Source: CAD feature listing. Evaluate the final solid. Frame: model axes, mm. A direction names the side the tool comes from. Give positions to 0.01 mm unless a question says otherwise; leave off trailing zeros. Write each loop counter-clockwise with the first axis right and the second up, starting at its lowest first coordinate (ties: lowest second). Pieces come first, ordered by that corner, then holes. Notation, with made-up numbers: (-39.5, 35) -> (-21.5, 35) arc R9 cw to (-21.5, 45) -> close; hole circle Ø5 at (-32, -31). An arc over 180 degrees is marked (long way). Write item = value, one per line.
from build123d import *

# Parameters (mm, degrees)
SKETCH1_W           = 12.7
SKETCH1_H           = 25.4
BOSS_EXTRUDE1_DEPTH = 50.8
SKETCH1_3_W         = 12.7
SKETCH1_3_H         = 25.4
BOSS_EXTRUDE2_DEPTH = 127
SKETCH2_R           = 19.05
SKETCH2_R_2         = 6.35
BOSS_EXTRUDE3_DEPTH = 12.7
BOSS_EXTRUDE4_START = -6.35
BOSS_EXTRUDE4_DEPTH = 19.05


with BuildPart() as part:
    # Sketch1 → Boss-Extrude1 (new body)
    with BuildSketch(Plane.XY):
        with BuildLine():
            Line((-38.1, -12.7), (-49.186888497, -12.7))
            ThreePointArc((-49.186888497, -12.7), (0, -50.8), (49.186888497, -12.7))
            Line((49.186888497, -12.7), (38.1, -12.7))
            Line((38.1, -12.7), (38.1, 12.7))
            Line((38.1, 12.7), (49.186888497, 12.7))
            ThreePointArc((49.186888497, 12.7), (0, 50.8), (-49.186888497, 12.7))
            Line((-49.186888497, 12.7), (-38.1, 12.7))
            Line((-38.1, 12.7), (-38.1, -12.7))
        make_face()
        Rectangle(SKETCH1_W, SKETCH1_H, mode=Mode.SUBTRACT)
    extrude(amount=-BOSS_EXTRUDE1_DEPTH)

    # Sketch1_3 → Boss-Extrude2 (add)
    with BuildSketch(Plane.XY):
        Rectangle(SKETCH1_3_W, SKETCH1_3_H)
    extrude(amount=-BOSS_EXTRUDE2_DEPTH)

    # Sketch2 → Boss-Extrude3 (add)
    with BuildSketch(Plane(origin=(6.35, 0, 0), x_dir=(0, 0, -1), z_dir=(1, 0, 0))):
        with Locations((127, 0)):
            Circle(SKETCH2_R)
        with Locations((127, 0)):
            Circle(SKETCH2_R_2, mode=Mode.SUBTRACT)
    extrude(amount=-BOSS_EXTRUDE3_DEPTH)

    # Sketch2_2 → Boss-Extrude4 (add, symmetric)
    with BuildSketch(Plane(origin=(6.35, 0, 0), x_dir=(0, 0, -1), z_dir=(1, 0, 0)).offset(BOSS_EXTRUDE4_START)):
        with BuildLine():
            ThreePointArc((127, -6.35), (131.490128061, -4.490128061), (133.35, 0))
            ThreePointArc((133.35, 0), (131.490128061, 4.490128061), (127, 6.35))
            Line((127, 6.35), (127, -6.35))
        make_face()
        with BuildLine():
            Line((127, -6.35), (127, 6.35))
            ThreePointArc((127, 6.35), (120.65, 0), (127, -6.35))
        make_face()
    extrude(amount=BOSS_EXTRUDE4_DEPTH, both=True)


solid = part.part
1) Material intervals for L1, parallel to Z at x = -6, y = 34; L2, parallel to Y at x = 3, z = -77; L3, parallel to X at y = 1.5, z = -11.5, sorted ascending.
Computed:
L1 = -50.8 to 0
L2 = -12.7 to 12.7
L3 = -38.1 to 38.1
2) Cut plane C-C (y = -17). Return the cut outline in (x, z), then the cut area to 3 significant figures.
Computed:
outline = (-47.87, -50.8) -> (47.87, -50.8) -> (47.87, 0) -> (-47.87, 0) -> close; (-6.35, -135.6) -> (6.35, -135.6) -> (6.35, -118.4) -> (-6.35, -118.4) -> close
area = 5,080 mm²
3) Contact query for flat-ended pins moving along their axis: pin 1 (14 mm diameter, centred on x = 0.5, z = -81.5, fed in from -Y); pin 2 (14 mm diameter, centred on y = 1, z = -127.5, fed in from -X); pin 3 (9 mm diameter, centred on x = 45, z = -34, fed in from +Y); pin 4 (10 mm diameter, centred on y = -26, z = -115.5, fed in from +X). Output: stop coordinate, or through.
Computed:
pin_1 = -12.7
pin_2 = -19.05
pin_3 = 30.67
pin_4 = through
4) Cut plane D-D (y = -43.5). Return the cut outline in (x, z), then the cut area to 3 significant figures.
Computed:
outline = (-26.24, -50.8) -> (26.24, -50.8) -> (26.24, 0) -> (-26.24, 0) -> close
area = 2,670 mm²
5) Draft query along Z for faces 1 (the flat face through (44, 12.7, -25)), 2 (the flat face through (6.35, 0, -98)), 3 (the flat face through (-1, 1, 0)), 4 (the flat face through (-6.35, 0, -98)). Return one class per face: pulls with the +Z half, pulls with the -Z half, needs draft (parallel to the pull), parting line crosses it, or undercut.
Computed:
face_1 = needs draft
face_2 = undercut
face_3 = pulls with the +Z half
face_4 = undercut
6) Cut plane B-B (z = -33). Return the cut outline in (x, y), then the cut area to 3 significant figures.
Computed:
outline = (-49.19, -12.7) arc R50.8 ccw to (49.19, -12.7) -> (38.1, -12.7) -> (38.1, 12.7) -> (49.19, 12.7) arc R50.8 ccw to (-49.19, 12.7) -> (-38.1, 12.7) -> (-38.1, -12.7) -> close
area = 7,490 mm²
7) Access query for faces 5 (the flat face through (38.1, 0, -25)), 6 (the flat face through (-44, 12.7, -25)), 7 (the flat face through (0, 12.7, -81)), 8 (the flat face through (19.05, 0, -127)). Directions: +Z, -Z, +X, -X, +Y, -Y. A direction counts if a zero-diameter tool reaches every point of the face in a straight line with its end or side. Return the directions, or none.
Computed:
face_5 = +Z, -Z, +X
face_6 = +Z, -Z, -X
face_7 = +X, -X, +Y
face_8 = -Z, +X, +Y, -Y
8) Cut plane A-A (x = -13.5). Return the cut outline in (y, z).
Computed:
outline = (-48.97, -50.8) -> (48.97, -50.8) -> (48.97, 0) -> (-48.97, 0) -> close; circle Ø12.7 at (0, -127)
